from build123d import *

# Parameters (mm, degrees)
F0_W      = 35
F0_H      = 60
F1_DEPTH  = 45
F2_W      = 25
F2_H      = 40
F2_H_2    = 60
F3_DEPTH  = 65
F4_W      = 10
F4_H      = 30
F5_DEPTH  = 45
F7_DEPTH  = 100
F9_DEPTH  = 40
F11_DEPTH = 85


with BuildPart() as f1:
    # F0 (on Front) → F1 (new body)
    with BuildSketch(Plane.XZ):
        with Locations((-17.5, 30)):
            Rectangle(F0_W, F0_H)
    extrude(amount=F1_DEPTH)

    # F2 (on face) → F3 (join)
    with BuildSketch(Plane(origin=(0, 0, 0), x_dir=(-1, 0, 0), z_dir=(0, 1, 0))):
        with Locations((22.5, 80)):
            Rectangle(F2_W, F2_H)
        with Locations((22.5, 30)):
            Rectangle(F2_W, F2_H_2)
    extrude(amount=F3_DEPTH)

    # F4 (on face) → F5 (cut)
    with BuildSketch(Plane(origin=(0, 65, 0), x_dir=(-1, 0, 0), z_dir=(0, 1, 0))):
        with Locations((15, 45)):
            Rectangle(F4_W, F4_H)
    extrude(amount=-F5_DEPTH, mode=Mode.SUBTRACT)

    # F6 (on face) → F7 (cut)
    with BuildSketch(Plane.XY.offset(100)):
        Polygon((-10, 45), (-10, 65), (-35, 65), align=None)
    extrude(amount=-F7_DEPTH, mode=Mode.SUBTRACT)

    # F8 (on face) → F9 (join)
    with BuildSketch(Plane.XY.offset(60)):
        Polygon((-35, -30), (-35, -45), (-10, -45), align=None)
    extrude(amount=F9_DEPTH)

    # F10 (on face) → F11 (cut)
    with BuildSketch(Plane.XY.offset(100)):
        Polygon((-35, 15), (-35, 0), (-11, 0), align=None)
    extrude(amount=-F11_DEPTH, mode=Mode.SUBTRACT)


solid = f1.part
Model file for the job. Use its own axes, mm. A direction names the side the tool comes from. Coordinates: 2 decimals unless noted, no trailing zeros. Write each loop counter-clockwise with the first axis right and the second up, starting at its lowest first coordinate (ties: lowest second). Pieces come first, ordered by that corner, then holes. Notation, with made-up numbers: (73, -17.75) -> (79, -17.75) arc R8 ccw to (79, -13.75) -> close; hole circle Ø4 at (10, 69). An arc over 180 degrees is marked (long way). One line per item, written item: value. Start each with the question number.
1) Slice it at D-D on z = 39.5. Write the cut outline in (x, y).
2) Slice it at B-B on x = -17. Write the cut outline in (y, z).
3) Slice it at A-A on z = 89.5. Write the cut outline in (x, y).
4) Which spindle directions (+Z, -Z, +X, -X, +Y, -Y) get a long thin tool onto all of the face, cutting with end or side? Do faces 5 (the face through (-18, -22, 60)), 6 (the face through (-15, 33, 30)), 7 (the face through (-22.832, 7.395, 58.095)), 8 (the face through (-10, 17, 51)), 9 (the face through (-35, 23, 38)). Say none if no direction does.
5) Flat gauge pins, fed straight in: pin 1 Ø8 at (x, z) = (-13.5, 14.5) entering from +Y; pin 2 Ø10 at (x, z) = (-7.5, 11.5) entering from +Y; pin 3 Ø12 at (y, z) = (38.5, 63.5) entering from +X; pin 4 Ø3 at (y, z) = (-23.5, 35) entering from +X. Where does each tip first touch, or does it go through?
6) Slice it at C-C on y = 47. Write the cut outline in (x, z).
7) Pull direction Y, two halves, no side cores. Call faces 1 (the face through (-22, 32, 100)), 2 (the face through (-22.33, -37.6, 79.72)), 3 (the face through (-5, 0, 30)), 4 (the face through (-22, -45, 49)): +Y half, -Y half, draft (parallel to the pull), parting line (faces both ways), or undercut.
8) Probe probe 1 along Z at (x, y) = (-8, -37); probe 2 along Z at (x, y) = (-14.5, 24.5); probe 3 along X at (y, z) = (39, 41.5). List the from-to ranges inside material, lowest first.
Answers follow:
1. outline: (-35, -45) -> (0, -45) -> (0, 0) -> (-10, 0) -> (-10, 20) -> (-20, 20) -> (-20, 53) -> (-35, 65) -> (-35, 15) -> (-11, 0) -> (-35, 0) -> close
2. outline: (-45, 0) -> (50.6, 0) -> (50.6, 30) -> (20, 30) -> (20, 60) -> (50.6, 60) -> (50.6, 100) -> (3.75, 100) -> (3.75, 15) -> (0, 15) -> (0, 60) -> (-40.8, 60) -> (-40.8, 100) -> (-45, 100) -> close
3. outline: (-35, -45) -> (-10, -45) -> (-35, -30) -> close; (-35, 15) -> (-11, 0) -> (-10, 0) -> (-10, 45) -> (-35, 65) -> close
4. face 5: +Z, +X
4. face 6: +X, +Y
4. face 7: +Z, -X
4. face 8: +Z, -Z, +X, +Y
4. face 9: +Z, -Z, -X, +Y, -Y
5. pin 1: y = 51
5. pin 2: y = 47
5. pin 3: x = -10
5. pin 4: x = 0
6. outline: (-35, 0) -> (-12.5, 0) -> (-12.5, 30) -> (-20, 30) -> (-20, 60) -> (-12.5, 60) -> (-12.5, 100) -> (-35, 100) -> close
7. face 1: draft
7. face 2: undercut
7. face 3: +Y half
7. face 4: -Y half
8. probe 1: 0 to 60
8. probe 2: 0 to 30, 60 to 100
8. probe 3: -35 to -20
